Here's how the part is built. I have some questions about the finished solid (model axes, mm). A direction names the side the tool comes from. Round coordinates to 2 decimals unless told otherwise and drop trailing zeros. Order: outer loops, then holes, each group sorted by start corner. A loop starts at its lowest first (then second) coordinate and runs counter-clockwise, first axis right, second up. Notation, with made-up numbers: (25, 29.5) -> (45, 29.5) arc R29 ccw to (45, 61.5) -> close; hole circle Ø9 at (73.25, -30.75). An arc over 180 degrees is marked (long way). Use a Markdown table: item, result. Add a question column.
(1) Thinking about a two-plate mould opening in X: for faces 3 (the face through (13.274, -1.479, 9.805)), 4 (the face through (-23.45, -1, 0)), 5 (the face through (23.45, -1, 0)), which applies, pulls with the +X half, pulls with the -X half, needs draft (parallel to the pull), parting line crosses it, or undercut?
(2) If I drill on probe 1 along X at (y, z) = (-2.1, 0.75) (3 decimals); probe 2 along Z at (x, y) = (-5, -0.3) (3 decimals); probe 3 along Z at (x, y) = (12.5, -1.8), over which ranges is the centre line in solid material (lowest first)?
(3) I want a section at A-A, the plane z = 4. Please give me the cut outline in (x, y) (3 decimals), then the cut area to 4 significant figures.
(4) On a 3-axis mill with a long thin cutter (end or side, diameter ignored), from which of +Z, -Z, +X, -X, +Y, -Y can I reach the whole of each face in a straight line? I mean faces 1 (the face through (0, 0, -13)), 2 (the face through (-13.305, -1.479, 9.774)). Say none if no direction works.
(5) I want a section at C-C, the plane y = -2. Please give me the cut outline in (x, z) (3 decimals), then the cut area to 3 significant figures.
(6) I want a section at B-B, the plane x = -7.5. Please give me the cut outline in (y, z) (3 decimals), then the cut area to 4 significant figures.
from build123d import *

# Parameters (mm, degrees)
F0_W     = 46.9
F0_H     = 29.9
F1_DEPTH = 3


with BuildPart() as f1:
    # F0 (on Front) → F1 (new body)
    with BuildSketch(Plane.XZ):
        Rectangle(F0_W, F0_H)
        with BuildLine():
            Line((11.875, -10.375), (-11.875, -10.375))
            ThreePointArc((-11.875, -10.375), (-13.289214, -9.789214), (-13.875, -8.375))
            Line((-13.875, -8.375), (-13.875, 8.375))
            ThreePointArc((-13.875, 8.375), (-13.289214, 9.789214), (-11.875, 10.375))
            Line((-11.875, 10.375), (11.875, 10.375))
            ThreePointArc((11.875, 10.375), (13.289214, 9.789214), (13.875, 8.375))
            Line((13.875, 8.375), (13.875, -8.375))
            ThreePointArc((13.875, -8.375), (13.289214, -9.789214), (11.875, -10.375))
        make_face(mode=Mode.SUBTRACT)
    extrude(amount=F1_DEPTH)


solid = f1.part
Taken from the geometry:
| question | item | result |
|---|---|---|
| 1 | face 3 | undercut |
| 1 | face 4 | pulls with the -X half |
| 1 | face 5 | pulls with the +X half |
| 2 | probe 1 | x = -23.45 to -13.875, 13.875 to 23.45 |
| 2 | probe 2 | z = -14.95 to -10.375, 10.375 to 14.95 |
| 2 | probe 3 | z = -14.95 to -10.27, 10.27 to 14.95 |
| 3 | outline | (-23.45, -3) -> (-13.875, -3) -> (-13.875, 0) -> (-23.45, 0) -> close; (13.875, -3) -> (23.45, -3) -> (23.45, 0) -> (13.875, 0) -> close |
| 3 | area | 57.45 mm2 |
| 4 | face 1 | +Z, -Z, +X, -X, +Y |
| 4 | face 2 | +Y, -Y |
| 5 | outline | (-23.45, -14.95) -> (23.45, -14.95) -> (23.45, 14.95) -> (-23.45, 14.95) -> close; hole (-13.875, -8.375) arc R2 ccw to (-11.875, -10.375) -> (11.875, -10.375) arc R2 ccw to (13.875, -8.375) -> (13.875, 8.375) arc R2 ccw to (11.875, 10.375) -> (-11.875, 10.375) arc R2 ccw to (-13.875, 8.375) -> close |
| 5 | area | 830 mm2 |
| 6 | outline | (-3, -14.95) -> (0, -14.95) -> (0, -10.375) -> (-3, -10.375) -> close; (-3, 10.375) -> (0, 10.375) -> (0, 14.95) -> (-3, 14.95) -> close |
| 6 | area | 27.45 mm2 |
